from build123d import *

# Parameters (mm, degrees)
SKETCH1_W                      = 150
SKETCH1_H                      = 60
BOSS_EXTRUDE1_DEPTH            = 3.175
CONVERT_SOLID1_OUTLINE_W       = 150
CONVERT_SOLID1_OUTLINE_H       = 60
CONVERT_SOLID1_DEPTH           = 0.05
SKETCHED_START                 = -30
SKETCHED_BEND1_DEPTH           = 60
SKETCHED_BEND1_2_DEPTH         = 60
SKETCH12_W                     = 13.513441401
SKETCH12_H                     = 61.735090191
CUT_EXTRUDE1_DEPTH             = 51.24
SKETCH13_R                     = 3.5
CUT_EXTRUDE2_DEPTH             = 10
SKETCH14_W                     = 60
SKETCH14_H                     = 3.125
BOSS_EXTRUDE2_DEPTH            = 3.5
M5_CLEARANCE_HOLE1_D           = 5.5
M5_CLEARANCE_HOLE1_DEPTH       = 10.1
M5_CLEARANCE_HOLE1_CSINK_D     = 5.55
M5_CLEARANCE_HOLE1_CSINK_ANGLE = 90
M5_CLEARANCE_HOLE1_TIP         = 1.652366702
M5_CLEARANCE_HOLE2_AT_2_COUNT  = 2
M5_CLEARANCE_HOLE2_AT_2_PITCH  = 30


# Read off the part's stored shape, not the designer's step: Convert-Solid1, Sketched Bend1
with BuildPart() as part:
    # Sketch1 → Boss-Extrude1 (new body)
    with BuildSketch(Plane(origin=(0, 0, 0), x_dir=(1, 0, 0), z_dir=(0, 1, 0))):
        Rectangle(SKETCH1_W, SKETCH1_H)
    extrude(amount=BOSS_EXTRUDE1_DEPTH)

    # Convert-Solid1 outline → Convert-Solid1 (cut)
    with BuildSketch(Plane(origin=(0, 0, 0), x_dir=(1, 0, 0), z_dir=(0, 1, 0))):
        Rectangle(CONVERT_SOLID1_OUTLINE_W, CONVERT_SOLID1_OUTLINE_H)
    extrude(amount=CONVERT_SOLID1_DEPTH, mode=Mode.SUBTRACT)

    # Sketched Bend1 outline → Sketched Bend1 (cut)
    with BuildSketch(Plane.XY.offset(SKETCHED_START)):
        with BuildLine():
            ThreePointArc((3.72475079, 0.05), (0.586030908, 0.886777026), (-1.719569645, 3.175))
            Line((-1.719569645, 3.175), (-75, 3.175))
            Line((-75, 3.175), (-75, 0.05))
            Line((-75, 0.05), (3.72475079, 0.05))
        make_face()
    extrude(amount=SKETCHED_BEND1_DEPTH, mode=Mode.SUBTRACT)

    # Sketched Bend1 2 outline → Sketched Bend1 2 (add)
    with BuildSketch(Plane.XY.offset(SKETCHED_START)):
        with BuildLine():
            Line((0.54475079, 77.63024921), (-2.58024921, 77.63024921))
            Line((-2.58024921, 77.63024921), (-2.58024921, 6.355))
            ThreePointArc((-2.58024921, 6.355), (-2.361276869, 4.707792567), (-1.719569645, 3.175))
            Line((-1.719569645, 3.175), (3.72475079, 3.175))
            ThreePointArc((3.72475079, 3.175), (1.476151226, 4.106400436), (0.54475079, 6.355))
            Line((0.54475079, 6.355), (0.54475079, 77.63024921))
        make_face()
    extrude(amount=SKETCHED_BEND1_2_DEPTH)

    # Sketch12 → Cut-Extrude1 (cut)
    with BuildSketch(Plane(origin=(0, 79.093833736, 0), x_dir=(1, 0, 0), z_dir=(0, 1, 0))):
        with Locations((-1.719442409, -0.853480509)):
            Rectangle(SKETCH12_W, SKETCH12_H)
    extrude(amount=-CUT_EXTRUDE1_DEPTH, mode=Mode.SUBTRACT)

    # Sketch13 → Cut-Extrude2 (cut)
    with BuildSketch(Plane(origin=(0, 3.175, 0), x_dir=(1, 0, 0), z_dir=(0, 1, 0))):
        with Locations(Location((50, 0, 0), (0, 0, 270))):
            Circle(SKETCH13_R)
    extrude(amount=-CUT_EXTRUDE2_DEPTH, mode=Mode.SUBTRACT)

    # Sketch14 → Boss-Extrude2 (add)
    with BuildSketch(Plane(origin=(75, 0, 0), x_dir=(0, 0, -1), z_dir=(1, 0, 0))):
        with Locations((0, 1.6125)):
            Rectangle(SKETCH14_W, SKETCH14_H)
    extrude(amount=BOSS_EXTRUDE2_DEPTH)

    # M5 Clearance Hole1
    with Locations(Plane(origin=(0, 3.175, 0), x_dir=(1, 0, 0), z_dir=(0, 1, 0))):
        with Locations((30, 20), (70, 20), (70, -20), (30, -20), (50, 20), (50, -20), (70, 0), (30, 0)):
            CounterSinkHole(M5_CLEARANCE_HOLE1_D / 2, M5_CLEARANCE_HOLE1_CSINK_D / 2, depth=M5_CLEARANCE_HOLE1_DEPTH, counter_sink_angle=M5_CLEARANCE_HOLE1_CSINK_ANGLE)
            with Locations((0, 0, -(M5_CLEARANCE_HOLE1_DEPTH + M5_CLEARANCE_HOLE1_TIP / 2))):  # 118° drill point
                Cone(0, M5_CLEARANCE_HOLE1_D / 2, M5_CLEARANCE_HOLE1_TIP, mode=Mode.SUBTRACT)

    # Sketch21 → M5 Clearance Hole2 (revolve, cut)
    with BuildSketch(Plane(origin=(0.54475079, 7.853833736, 15), x_dir=(0, 0, -1), z_dir=(0, 1, 0))):
        Polygon((0, 0), (0, 11.752366702), (2.75, 10.1), (2.75, 0.025), (2.775, 0), align=None)
    m5_clearance_hole2 = revolve(axis=Axis((6.89475079, 7.853833736, 15), (-1, 0, 0)), mode=Mode.SUBTRACT)

    # M5 Clearance Hole2 at 2: M5 Clearance Hole2 ×2
    with Locations(*[(0, 0, -i * M5_CLEARANCE_HOLE2_AT_2_PITCH) for i in range(1, M5_CLEARANCE_HOLE2_AT_2_COUNT)]):
        add(m5_clearance_hole2, mode=Mode.SUBTRACT)


solid = part.part
Model file for the job. Use its own axes, mm. A direction names the side the tool comes from. Round coordinates to 2 decimals unless told otherwise and drop trailing zeros. Loops run counter-clockwise (first coordinate to the right, second up) from the corner with the lowest first, then second, coordinate; pieces in that order, holes last. Notation, with made-up numbers: (-15, -12.75) -> (33, -12.75) arc R14 ccw to (33, 11.25) -> close; hole circle Ø10 at (43.25, 56.5). An arc over 180 degrees is marked (long way). Answer as CSV lines item,"result". Start each with the question number.
1) Pin check, flat tips, straight feed: P1, Ø9, axis at y = 7.85, z = -15, coming from the -X side; P2, Ø2, axis at y = 10, z = 20.5, coming from the +X side; P3, Ø12, axis at x = 15.5, z = 1.5, coming from the +Y side (3 decimals); P4, Ø1, axis at y = 5.5, z = 14.5, coming from the -X side. Stop position of each tip, or through.
2) Slice it at D-D (x = 30). List the corners of the cut face in (y, z) (3 decimals), plus the area to 3 significant figures.
3) Mould opens along X. For faces 1 (the face through (41, 0.05, 0)), 2 (the face through (78.5, 2, 0)), 3 (the face through (32.747, 1.578, 19.879)) say: +X half, -X half, draft (parallel to the pull), parting line (faces both ways), or undercut.
4) Slice it at A-A (x = 50). List the corners of the cut face in (y, z) (3 decimals).
5) Slice it at B-B (z = 0). List the corners of the cut face in (x, y) (3 decimals).
6) Tool access for faces 4 (the face through (-1.009, 7.733, -12.253)), 5 (the face through (72.747, 1.578, -0.121)): list every direction of +Z, -Z, +X, -X, +Y, -Y with a clear straight run to the whole face (end or side of a thin tool).
7) Slice it at C-C (z = -7.5). List the corners of the cut face in (x, y) (3 decimals), plus the area to 3 significant figures.
8) Probe line 1 along Z through (x, y) = (30, 2.2); line 2 along X through (y, z) = (1.3, -20); line 3 along X through (y, z) = (2.15, -20). List the from-to ranges inside material, lowest first.
Filled in:
1,P1,"stops at x = -2.58"
1,P2,"stops at x = 0.54"
1,P3,"stops at y = 3.175"
1,P4,"stops at x = -2.49"
2,outline,"(0.05, -30) -> (3.175, -30) -> (3.175, -22.775) -> (3.15, -22.75) -> (0.05, -22.75) -> close; (0.05, -17.25) -> (3.15, -17.25) -> (3.175, -17.225) -> (3.175, -2.775) -> (3.15, -2.75) -> (0.05, -2.75) -> close; (0.05, 2.75) -> (3.15, 2.75) -> (3.175, 2.775) -> (3.175, 17.225) -> (3.15, 17.25) -> (0.05, 17.25) -> close; (0.05, 22.75) -> (3.15, 22.75) -> (3.175, 22.775) -> (3.175, 30) -> (0.05, 30) -> close"
2,area,"136 mm2"
3,face 1,"draft"
3,face 2,"+X half"
3,face 3,"undercut"
4,outline,"(0.05, -30) -> (3.175, -30) -> (3.175, -22.775) -> (3.15, -22.75) -> (0.05, -22.75) -> close; (0.05, -17.25) -> (3.15, -17.25) -> (3.175, -17.225) -> (3.175, -3.5) -> (0.05, -3.5) -> close; (0.05, 3.5) -> (3.175, 3.5) -> (3.175, 17.225) -> (3.15, 17.25) -> (0.05, 17.25) -> close; (0.05, 22.75) -> (3.15, 22.75) -> (3.175, 22.775) -> (3.175, 30) -> (0.05, 30) -> close"
5,outline,"(-2.58, 6.355) arc R6.305 ccw to (3.725, 0.05) -> (27.25, 0.05) -> (27.25, 3.15) -> (27.225, 3.175) -> (3.725, 3.175) arc R3.18 cw to (0.545, 6.355) -> (0.545, 27.854) -> (-2.58, 27.854) -> close; (32.75, 0.05) -> (46.5, 0.05) -> (46.5, 3.175) -> (32.775, 3.175) -> (32.75, 3.15) -> close; (53.5, 0.05) -> (67.25, 0.05) -> (67.25, 3.15) -> (67.225, 3.175) -> (53.5, 3.175) -> close; (72.75, 0.05) -> (78.5, 0.05) -> (78.5, 3.175) -> (72.775, 3.175) -> (72.75, 3.15) -> close"
6,face 4,"-X"
6,face 5,"+Y, -Y"
7,outline,"(-2.58, 6.355) arc R6.305 ccw to (3.725, 0.05) -> (78.5, 0.05) -> (78.5, 3.175) -> (3.725, 3.175) arc R3.18 cw to (0.545, 6.355) -> (0.545, 27.854) -> (-2.58, 27.854) -> close"
7,area,"324 mm2"
8,line 1,"z = -30 to -22.75, -17.25 to -2.75, 2.75 to 17.25, 22.75 to 30"
8,line 2,"x = -0.04 to 27.25, 32.75 to 47.25, 52.75 to 67.25, 72.75 to 78.5"
8,line 3,"x = -0.97 to 27.25, 32.75 to 47.25, 52.75 to 67.25, 72.75 to 78.5"
